from build123d import *

# Parameters (mm, degrees)
SKETCH2_W            = 43
SKETCH2_H            = 23
SKETCH2_R            = 1.25
BOSS_EXTRUDE1_DEPTH  = 13
FILLET1_R            = 1
BOSS_EXTRUDE2_DEPTH  = 16
BOSS_EXTRUDE3_DEPTH  = 15
SKETCH5_R            = 0.625
BOSS_EXTRUDE4_DEPTH  = 5
FILLET2_R            = 3
SKETCH6_R            = 3.5
BOSS_EXTRUDE5_DEPTH  = 4
SKETCH7_R            = 1
BOSS_EXTRUDE7_DEPTH  = 11
SKETCH8_R            = 1.25
BOSS_EXTRUDE8_DEPTH  = 5
BOSS_EXTRUDE9_START  = 9
BOSS_EXTRUDE9_DEPTH  = 9
SKETCH10_R           = 2
BOSS_EXTRUDE10_DEPTH = 2


with BuildPart() as part:
    # Sketch2 → Boss-Extrude1 (new body)
    with BuildSketch(Plane(origin=(0, 0, 0), x_dir=(1, 0, 0), z_dir=(0, 1, 0))):
        with Locations((21.5, 11.5)):
            Rectangle(SKETCH2_W, SKETCH2_H)
        with Locations(Location((2.25, 20.75, 0), (0, 0, 90))):
            Circle(SKETCH2_R, mode=Mode.SUBTRACT)
        with Locations(Location((40.75, 20.75, 0), (0, 0, 90))):
            Circle(SKETCH2_R, mode=Mode.SUBTRACT)
        with Locations(Location((40.75, 2.25, 0), (0, 0, 90))):
            Circle(SKETCH2_R, mode=Mode.SUBTRACT)
        with Locations(Location((2.25, 2.25, 0), (0, 0, 90))):
            Circle(SKETCH2_R, mode=Mode.SUBTRACT)
    extrude(amount=BOSS_EXTRUDE1_DEPTH)

    # Fillet1
    fillet1_edges = [part.edges().sort_by_distance(p)[0] for p in [
        (0, 6.5, -23),
        (43, 6.5, -23),
        (43, 6.5, 0),
        (0, 6.5, 0),
    ]]
    fillet(fillet1_edges, radius=FILLET1_R)

    # Sketch3 → Boss-Extrude2 (add)
    with BuildSketch(Plane(origin=(0, 13, 0), x_dir=(1, 0, 0), z_dir=(0, 1, 0))):
        with BuildLine():
            Line((16, 19.5), (16, 3.5))
            ThreePointArc((16, 3.5), (8, 0), (0, 3.5))
            Line((0, 3.5), (0, 19.5))
            ThreePointArc((0, 19.5), (8, 23), (16, 19.5))
        make_face()
    extrude(amount=BOSS_EXTRUDE2_DEPTH)

    # Sketch4 → Boss-Extrude3 (add)
    with BuildSketch(Plane(origin=(0, 29, 0), x_dir=(1, 0, 0), z_dir=(0, 1, 0))):
        with BuildLine():
            Line((1, 18.5), (1, 4.5))
            ThreePointArc((1, 4.5), (8, 1.600505063), (15, 4.5))
            Line((15, 4.5), (15, 18.5))
            ThreePointArc((15, 18.5), (8, 21.399494937), (1, 18.5))
        make_face()
    extrude(amount=BOSS_EXTRUDE3_DEPTH)

    # Sketch5 → Boss-Extrude4 (add)
    with BuildSketch(Plane(origin=(0, 44, 0), x_dir=(1, 0, 0), z_dir=(0, 1, 0))):
        with Locations(Location((8, 11.5, 0), (0, 0, 90))):
            Circle(SKETCH5_R)
    extrude(amount=BOSS_EXTRUDE4_DEPTH)

    # Fillet2
    # the kernel refuses this fillet: 3 mm, written as the material it takes off along each edge
    with BuildSketch(Plane(origin=(8, 44, -11.5), x_dir=(0.5117233691003439, 0, 0.8591502741177431), z_dir=(-0.8591502741177431, 0, 0.5117233691003439))) as fillet2_piece_1:
        with BuildLine():
            CenterArc((9.899494937 - FILLET2_R, -FILLET2_R), FILLET2_R, 0, 90)
            Line((9.899494937 - FILLET2_R, 0), (9.899494937 - FILLET2_R, FILLET2_R * 0.02))
            Line((9.899494937 - FILLET2_R, FILLET2_R * 0.02), (9.899494937 + FILLET2_R * 0.02, FILLET2_R * 0.02))
            Line((9.899494937 + FILLET2_R * 0.02, FILLET2_R * 0.02), (9.899494937 + FILLET2_R * 0.02, -FILLET2_R))
            Line((9.899494937 + FILLET2_R * 0.02, -FILLET2_R), (9.899494937, -FILLET2_R))
        make_face()
    revolve(axis=Axis((8, 44, -11.5), (0, 1, 0)), revolution_arc=298.442618359, mode=Mode.SUBTRACT)
    with BuildSketch(Plane(origin=(8, 44, -11.5), x_dir=(-0.5117233691003458, 0, -0.859150274117742), z_dir=(0.859150274117742, 0, -0.5117233691003458))) as fillet2_piece_2:
        with BuildLine():
            CenterArc((9.899494937 - FILLET2_R, -FILLET2_R), FILLET2_R, 0, 90)
            Line((9.899494937 - FILLET2_R, 0), (9.899494937 - FILLET2_R, FILLET2_R * 0.02))
            Line((9.899494937 - FILLET2_R, FILLET2_R * 0.02), (9.899494937 + FILLET2_R * 0.02, FILLET2_R * 0.02))
            Line((9.899494937 + FILLET2_R * 0.02, FILLET2_R * 0.02), (9.899494937 + FILLET2_R * 0.02, -FILLET2_R))
            Line((9.899494937 + FILLET2_R * 0.02, -FILLET2_R), (9.899494937, -FILLET2_R))
        make_face()
    revolve(axis=Axis((8, 44, -11.5), (0, 1, 0)), revolution_arc=298.442618359, mode=Mode.SUBTRACT)

    # Sketch6 → Boss-Extrude5 (add)
    with BuildSketch(Plane(origin=(0, 13, 0), x_dir=(1, 0, 0), z_dir=(0, 1, 0))):
        with Locations(Location((31.75, 11.5, 0), (0, 0, 90))):
            Circle(SKETCH6_R)
    extrude(amount=BOSS_EXTRUDE5_DEPTH)

    # Sketch7 → Boss-Extrude7 (add)
    with BuildSketch(Plane(origin=(0, 17, 0), x_dir=(1, 0, 0), z_dir=(0, 1, 0))):
        with BuildLine():
            Line((29.75, 13.387458609), (33.75, 13.387458609))
            ThreePointArc((33.75, 13.387458609), (34.5, 11.5), (33.75, 9.612541391))
            Line((33.75, 9.612541391), (29.75, 9.612541391))
            ThreePointArc((29.75, 9.612541391), (29, 11.5), (29.75, 13.387458609))
        make_face()
        with Locations(Location((31.75, 11.5, 0), (0, 0, 270))):
            Circle(SKETCH7_R, mode=Mode.SUBTRACT)
    extrude(amount=BOSS_EXTRUDE7_DEPTH)

    # Sketch8 → Boss-Extrude8 (add)
    # profile 1 of 2: a face of its own
    with BuildSketch(Plane(origin=(0, 13, 0), x_dir=(1, 0, 0), z_dir=(0, 1, 0))):
        with BuildLine():
            Line((-3.437113108, 13.75), (0, 13.75))
            Line((0, 13.75), (0, 9.25))
            Line((0, 9.25), (-3.437113108, 9.25))
            ThreePointArc((-3.437113108, 9.25), (-5.687113108, 11.5), (-3.437113108, 13.75))
        make_face()
        with Locations(Location((-3.437113108, 11.5, 0), (0, 0, 270))):
            Circle(SKETCH8_R, mode=Mode.SUBTRACT)
    # profile 2 of 2: a face of its own
    with BuildSketch(Plane(origin=(0, 13, 0), x_dir=(1, 0, 0), z_dir=(0, 1, 0))):
        with BuildLine():
            Line((16, 9.25), (19.44, 9.25))
            ThreePointArc((19.44, 9.25), (21.69, 11.5), (19.44, 13.75))
            Line((19.44, 13.75), (16, 13.75))
            Line((16, 13.75), (16, 9.25))
        make_face()
        with Locations(Location((19.44, 11.5, 0), (0, 0, 270))):
            Circle(SKETCH8_R, mode=Mode.SUBTRACT)
    extrude(amount=BOSS_EXTRUDE8_DEPTH)

    # Sketch9 → Boss-Extrude9 (add)
    with BuildSketch(Plane.XZ.offset(BOSS_EXTRUDE9_START)):
        with BuildLine():
            Line((33.75, -13.387458609), (29.75, -13.387458609))
            ThreePointArc((29.75, -13.387458609), (29, -11.5), (29.75, -9.612541391))
            Line((29.75, -9.612541391), (33.75, -9.612541391))
            ThreePointArc((33.75, -9.612541391), (34.5, -11.5), (33.75, -13.387458609))
        make_face()
    extrude(amount=-BOSS_EXTRUDE9_DEPTH)

    # Sketch10 → Boss-Extrude10 (add)
    with BuildSketch(Plane.XZ):
        with Locations(Location((20.75, -11.5, 0), (0, 0, 270))):
            Circle(SKETCH10_R)
    extrude(amount=BOSS_EXTRUDE10_DEPTH)


solid = part.part
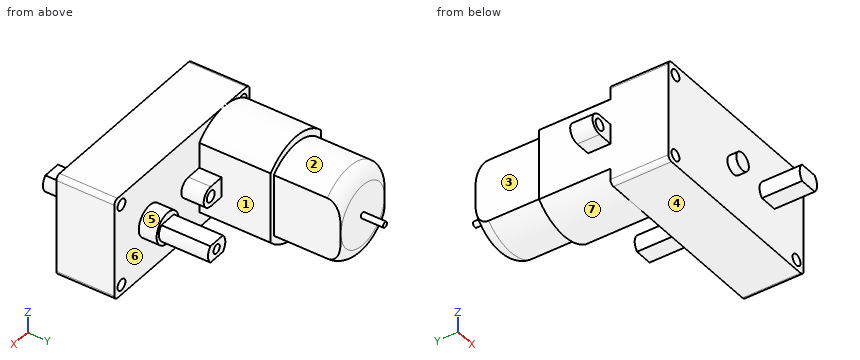
Model file for the job. Use its own axes, mm. Face numbers are marked on the shaded views. A direction names the side the tool comes from. Round coordinates to 2 decimals unless told otherwise and drop trailing zeros. Order: outer loops, then holes, each group sorted by start corner. A loop starts at its lowest first (then second) coordinate and runs counter-clockwise, first axis right, second up.
(1) Drill centre lines: line 1 (X direction, y = 25.5, z = -11.5); line 2 (X direction, y = 8.25, z = -20.75); line 3 (Z direction, x = 40.75, y = 8). Where is each one in solid material? Low to high.
(2) Band-saw the part on D-D (y = 1). List the corners of the cut face in (x, z), then the cut area to 3 significant figures.
(3) Pin check, flat tips, straight feed: pin 1 (5 mm diameter, centred on x = 11.5, z = -13, fed in from +Y); pin 2 (4.5 mm diameter, centred on x = 32.5, y = 24, fed in from -Z); pin 3 (1.1 mm diameter, centred on x = 31, z = -12, fed in from +Y). Stop position of each tip, or through.
(4) Pull direction X, two halves, no side cores. Call the marked faces 4, 5, 6 and 7: released by +X, released by -X, zero draft, split by the parting line, or undercut.
(5) Band-saw the part on C-C (x = 31.75). List the corners of the cut face in (y, z), then the cut area to 3 significant figures.
(6) Band-saw the part on B-B (y = 26.5). List the corners of the cut face in (x, z).
(7) 3-axis set-ups, long thin cutter, end or side, ignore diameter. For the marked faces 1, 2 and 3: which of +Z, -Z, +X, -X, +Y, -Y reach the whole face in a straight line?
(8) Band-saw the part on A-A (y = 14). List the corners of the cut face in (x, z), then the cut area to 3 significant figures.
Verdict:
1. line 1: x = 0 to 16, 29 to 30.75, 32.75 to 34.5
1. line 2: x = 0 to 1, 3.5 to 39.5, 42 to 43
1. line 3: z = -23 to -22, -19.5 to -3.5, -1 to 0
2. outline: (0, -22) arc R1 ccw to (1, -23) - (42, -23) arc R1 ccw to (43, -22) - (43, -1) arc R1 ccw to (42, 0) - (1, 0) arc R1 ccw to (0, -1) - close; hole circle Ø2.5 at (2.25, -20.75); hole circle Ø2.5 at (2.25, -2.25); hole circle Ø2.5 at (40.75, -20.75); hole circle Ø2.5 at (40.75, -2.25)
2. area: 969 mm2
3. pin 1: stops at y = 44
3. pin 2: stops at z = -13.39
3. pin 3: stops at y = 28
4. face 4: zero draft
4. face 5: undercut
4. face 6: undercut
4. face 7: split by the parting line
5. outline: (-9, -13.39) - (0, -13.39) - (0, -23) - (13, -23) - (13, -15) - (17, -15) - (17, -13.39) - (28, -13.39) - (28, -12.5) - (17, -12.5) - (17, -10.5) - (28, -10.5) - (28, -9.61) - (17, -9.61) - (17, -8) - (13, -8) - (13, 0) - (0, 0) - (0, -9.61) - (-9, -9.61) - close
5. area: 380 mm2
6. outline: (0, -19.5) arc R10.89 ccw to (16, -19.5) - (16, -3.5) arc R10.89 ccw to (0, -3.5) - close; (29.75, -13.39) - (33.75, -13.39) arc R2.75 ccw to (33.75, -9.61) - (29.75, -9.61) arc R2.75 ccw to start; hole circle Ø2 at (31.75, -11.5)
7. face 1: +Y
7. face 2: +Z, +Y
7. face 3: +Z, -Z, -X, +Y
8. outline: (-3.44, -13.75) - (0, -13.75) - (0, -19.5) arc R10.89 ccw to (16, -19.5) - (16, -13.75) - (19.44, -13.75) arc R2.25 ccw to (19.44, -9.25) - (16, -9.25) - (16, -3.5) arc R10.89 ccw to (0, -3.5) - (0, -9.25) - (-3.44, -9.25) arc R2.25 ccw to start; circle Ø7 at (31.75, -11.5); hole circle Ø2.5 at (-3.44, -11.5); hole circle Ø2.5 at (19.44, -11.5)
8. area: 409 mm2
